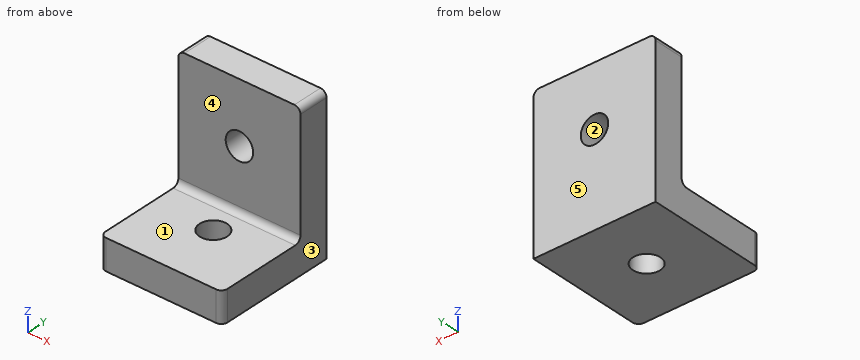
from build123d import *

# Parameters (mm, degrees)
F0_W     = 20
F0_H     = 15
F0_R     = 2.25
F1_DEPTH = 5
F0_H_2   = 5
F2_DEPTH = 25
F3_R     = 2.25
F4_DEPTH = 25
F5_R     = 1


with BuildPart() as f1:
    # F0 (on Top) → F1 (new body)
    with BuildSketch(Plane.XY):
        with Locations((0.344828, 7.5)):
            Rectangle(F0_W, F0_H)
        with Locations((0.344828, 10)):
            Circle(F0_R, mode=Mode.SUBTRACT)
    extrude(amount=F1_DEPTH)

    # F0 (on Top) → F2 (join)
    with BuildSketch(Plane.XY):
        with Locations((0.344828, 17.5)):
            Rectangle(F0_W, F0_H_2)
    extrude(amount=F2_DEPTH)

    # F3 (on face) → F4 (cut)
    with BuildSketch(Plane.XZ.offset(-15)):
        with Locations((0.344828, 15)):
            Circle(F3_R)
    extrude(amount=-F4_DEPTH, mode=Mode.SUBTRACT)

    # F5
    f5_edges = [f1.edges().sort_by_distance(p)[0] for p in [
        (-9.655172, 17.5, 25),
        (10.344828, 17.5, 25),
        (-9.655172, 0, 2.5),
        (10.344828, 0, 2.5),
        (0.344828, 15, 5),
    ]]
    fillet(f5_edges, radius=F5_R)


solid = f1.part
Model file for the job. Use its own axes, mm. Face numbers are marked on the shaded views. A direction names the side the tool comes from. Round coordinates to 2 decimals unless told otherwise and drop trailing zeros. Loops run counter-clockwise (first coordinate to the right, second up) from the corner with the lowest first, then second, coordinate; pieces in that order, holes last.
1. Band-saw the part on D-D, the plane y = 17.5. List the corners of the cut face in (x, z), and give its area (3 significant figures).
Check values:
outline: (-9.66, 0) - (10.34, 0) - (10.34, 24) arc R1 ccw to (9.34, 25) - (-8.66, 25) arc R1 ccw to (-9.66, 24) - close; hole circle Ø4.5 at (0.34, 15)
area: 484 mm2
2. Wall check: probe 1 along Z at (x, y) = (-7.75, 10.75); probe 2 along Y at (x, z) = (7.5, 10); probe 3 along Z at (x, y) = (1, 16.75). Give the ranges that are in metal, low to high.
Check values:
probe 1: z = 0 to 5
probe 2: y = 15 to 20
probe 3: z = 0 to 12.85, 17.15 to 25
3. Band-saw the part on C-C, the plane z = 4. List the corners of the cut face in (x, y), and give its area (3 significant figures).
Check values:
outline: (-9.66, 1) arc R1 ccw to (-8.66, 0) - (9.34, 0) arc R1 ccw to (10.34, 1) - (10.34, 20) - (-9.66, 20) - close; hole circle Ø4.5 at (0.34, 10)
area: 384 mm2
4. Tool access for the marked faces 4 and 5: list every direction of +Z, -Z, +X, -X, +Y, -Y with a clear straight run to the whole face (end or side of a thin tool).
Check values:
face 4: +Z, +X, -X, -Y
face 5: +Z, -Z, +X, -X, +Y
5. Drop flat-ended pins along their axis: P1, Ø3.5, axis at x = 0.34, y = 10, coming from the -Z side; P2, Ø7, axis at x = 3.5, y = 8, coming from the +Z side; P3, Ø12, axis at x = -2, z = 20.5, coming from the -Y side. Give the stop position or say it passes through.
Check values:
P1: passes through
P2: stops at z = 5
P3: stops at y = 15
6. Band-saw the part on B-B, the plane z = 15. List the corners of the cut face in (x, y).
Check values:
outline: (-9.66, 15) - (-1.91, 15) - (-1.91, 20) - (-9.66, 20) - close; (2.59, 15) - (10.34, 15) - (10.34, 20) - (2.59, 20) - close
7. Mould opens along Z. For the marked faces 1, 2 and 3 say: +Z half, -Z half, draft (parallel to the pull), parting line (faces both ways), or undercut.
Check values:
face 1: +Z half
face 2: undercut
face 3: draft
8. Band-saw the part on A-A, the plane y = 10. List the corners of the cut face in (x, z), and give its area (3 significant figures).
Check values:
outline: (-9.66, 0) - (-1.91, 0) - (-1.91, 5) - (-9.66, 5) - close; (2.59, 0) - (10.34, 0) - (10.34, 5) - (2.59, 5) - close
area: 77.5 mm2
